Design review of the part built by this model. Coordinates are the model's own, in mm. A direction names the side the tool comes from. Give positions to 0.01 mm unless a question says otherwise; leave off trailing zeros. Write each loop counter-clockwise with the first axis right and the second up, starting at its lowest first coordinate (ties: lowest second). Pieces come first, ordered by that corner, then holes. Notation, with made-up numbers: M -21,68 L -3,68 A16 ccw -3,98 Z; hole C -12.5,65 d10. An arc over 180 degrees is marked long. Answer in a Markdown table with one row per item.
```python
from build123d import *

# Parameters (mm, degrees)
SKETCH_1_R          = 3
EXTRUDE_1_DEPTH     = 10
CUT_EXTRUDE_1_DEPTH = 1


with BuildPart() as part:
    # 草圖1 → 填料-伸長1 (new body)
    with BuildSketch(Plane(origin=(0, 0, 0), x_dir=(1, 0, 0), z_dir=(0, 1, 0))):
        with BuildLine():
            Line((0, 35), (28.284271247, 35))
            ThreePointArc((28.284271247, 35), (42.718027977, 30.412414523), (51.854497287, 18.333333333))
            ThreePointArc((51.854497287, 18.333333333), (54.894534338, 3.404423566), (53.722406301, -11.785714286))
            ThreePointArc((53.722406301, -11.785714286), (46.722649239, -23.083874449), (34.186985828, -27.5))
            Line((34.186985828, -27.5), (21.650635095, -27.5))
            ThreePointArc((21.650635095, -27.5), (-33.071891388, -11.456439237), (0, 35))
        make_face()
        with Locations(Location((0, 0, 0), (0, 0, 270))):
            Circle(SKETCH_1_R, mode=Mode.SUBTRACT)
    extrude(amount=EXTRUDE_1_DEPTH)

    # 草圖2 → 除料-伸長1 (cut)
    with BuildSketch(Plane(origin=(0, 10, 0), x_dir=(1, 0, 0), z_dir=(0, 1, 0))):
        with BuildLine():
            Line((0, -10), (0, -11))
            ThreePointArc((0, -11), (11, 0), (0, 11))
            Line((0, 11), (0, 11.5))
            Line((0, 11.5), (-1, 10.5))
            Line((-1, 10.5), (0, 9.5))
            Line((0, 9.5), (0, 10))
            ThreePointArc((0, 10), (10, 0), (0, -10))
        make_face()
    extrude(amount=-CUT_EXTRUDE_1_DEPTH, mode=Mode.SUBTRACT)


solid = part.part
```
1) Add section A-A (z = 0). Write out the cut boundary in (x, y), and give its area (3 significant figures).
Geometry says:
| item | result |
|---|---|
| outline | M -35,0 L -3,0 L -3,10 L -35,10 Z; M 3,0 L 55,0 L 55,10 L 11,10 L 11,9 L 10,9 L 10,10 L 3,10 Z |
| area | 839 mm^2 |
2) Insertion check: P1, Ø5, axis at y = 7.5, z = 27.5, coming from the -X side; P2, Ø5, axis at x = 0, z = 0, coming from the -Y side; P3, Ø0.6, axis at y = 9.5, z = -11, coming from the -X side; P4, Ø5, axis at x = -9.5, y = 4, coming from the +Z side. Each pin has a flat end and moves straight along its axis. Give the tip position at first contact, or say it passes through.
Geometry says:
| item | result |
|---|---|
| P1 | x = -24.49 |
| P2 | through |
| P3 | x = -33.32 |
| P4 | z = 34.29 |
3) The part is to be moulded in two halves that separate along Z. For faces 1 (the face through (14, 5, -35)), 2 (the face through (11, 10, -8)), 3 (the face through (10, 9, -2)), say which applies: released by +Z, released by -Z, zero draft, split by the parting line, or undercut.
Geometry says:
| item | result |
|---|---|
| face 1 | released by -Z |
| face 2 | zero draft |
| face 3 | undercut |
4) Add section C-C (x = 8.5). Write out the cut boundary in (y, z), and give its area (3 significant figures).
Geometry says:
| item | result |
|---|---|
| outline | M 0,-35 L 10,-35 L 10,-6.98 L 9,-6.98 L 9,-5.27 L 10,-5.27 L 10,5.27 L 9,5.27 L 9,6.98 L 10,6.98 L 10,33.95 L 0,33.95 Z |
| area | 686 mm^2 |
5) For faces 4 (the face through (0.9, 4.93, 2.86)), 5 (the face through (28, 5, 27.5)), 6 (the face through (11, 9.5, 0.2)), list the 3-axis set-ups (+Z, -Z, +X, -X, +Y, -Y) from which the entire face can be reached by the end or side of a thin tool; tool diameter is ignored.
Geometry says:
| item | result |
|---|---|
| face 4 | +Y, -Y |
| face 5 | +Z, +X, +Y, -Y |
| face 6 | +Y |
6) Add section D-D (z = 19.5). Write out the cut boundary in (x, y).
Geometry says:
| item | result |
|---|---|
| outline | M -29.06,0 L 50.19,0 L 50.19,10 L -29.06,10 Z |
7) To check wall thickness, follow probe 1 along X at (y, z) = (6, 0); probe 2 along X at (y, z) = (7.5, 1); probe 3 along X at (y, z) = (7, -22.5). State the ranges of each line that lie inside material, in increasing order. Write a range as [from, to].
Geometry says:
| item | result |
|---|---|
| probe 1 | [-35, -3], [3, 55] |
| probe 2 | [-34.99, -2.83], [2.83, 54.99] |
| probe 3 | [-26.81, 49.93] |
8) Add section B-B (y = 1.5). Write out the cut boundary in (x, z), and give its area (3 significant figures).
Geometry says:
| item | result |
|---|---|
| outline | M 0,-35 L 28.28,-35 A25 ccw 51.85,-18.33 A55 ccw 53.72,11.79 A20 ccw 34.19,27.5 L 21.65,27.5 A35 ccw long Z; hole C 0,0 d6 |
| area | 5,160 mm^2 |
